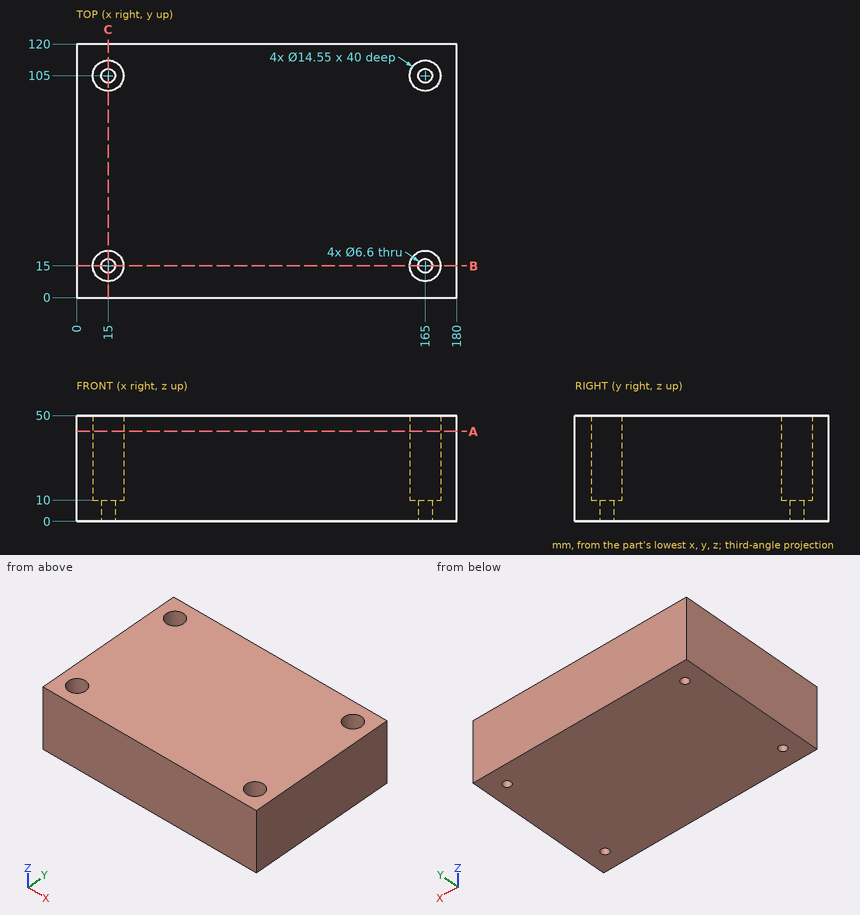
The drawing under review shows one solid part. Ordinate dimensions are in mm from its lowest x, y, z. Round coordinates to 2 decimals unless told otherwise and drop trailing zeros. Write each loop counter-clockwise with the first axis right and the second up, starting at its lowest first coordinate (ties: lowest second). Pieces come first, ordered by that corner, then holes. Notation, with made-up numbers: (2.25, 11) -> (40.25, 11) arc R25 ccw to (40.25, 41) -> close; hole circle Ø1 at (2, 17.25). An arc over 180 degrees is marked (long way). Put each result on its own line as item: value.
Q1. Clearance check with a flat-ended pin moving along its axis: pin 1 Ø4.5 at (x, y) = (15.5, 11.5) entering from +Z. State where the tip first meets the part, or that it passes through.
Determined:
pin 1: stops at z = 10
Q2. To check wall thickness, follow L1, parallel to Y at x = 15, z = 33 (3 decimals); L2, parallel to X at y = 15, z = 31.5 (3 decimals); L3, parallel to X at y = 105, z = 3.5. State the ranges of each line that lie inside material, in increasing order. Write a range as [from, to].
Determined:
L1: y = [0, 7.725], [22.275, 97.725], [112.275, 120]
L2: x = [0, 7.725], [22.275, 157.725], [172.275, 180]
L3: x = [0, 11.7], [18.3, 161.7], [168.3, 180]
Q3. Consider section B-B on y = 15. State the section outline as (x, z) points (3 decimals), and give its area (3 significant figures).
Determined:
outline: (0, 0) -> (11.7, 0) -> (11.7, 10) -> (7.725, 10) -> (7.725, 50) -> (0, 50) -> close; (18.3, 0) -> (161.7, 0) -> (161.7, 10) -> (157.725, 10) -> (157.725, 50) -> (22.275, 50) -> (22.275, 10) -> (18.3, 10) -> close; (168.3, 0) -> (180, 0) -> (180, 50) -> (172.275, 50) -> (172.275, 10) -> (168.3, 10) -> close
area: 7,700 mm^2
Q4. Consider section A-A on z = 42.5. State the section outline as (x, y) points (3 decimals), and give its area (3 significant figures).
Determined:
outline: (0, 0) -> (180, 0) -> (180, 120) -> (0, 120) -> close; hole circle Ø14.55 at (15, 15); hole circle Ø14.55 at (15, 105); hole circle Ø14.55 at (165, 15); hole circle Ø14.55 at (165, 105)
area: 20,900 mm^2
Q5. Consider section C-C on x = 15. State the section outline as (y, z) points (3 decimals).
Determined:
outline: (0, 0) -> (11.7, 0) -> (11.7, 10) -> (7.725, 10) -> (7.725, 50) -> (0, 50) -> close; (18.3, 0) -> (101.7, 0) -> (101.7, 10) -> (97.725, 10) -> (97.725, 50) -> (22.275, 50) -> (22.275, 10) -> (18.3, 10) -> close; (108.3, 0) -> (120, 0) -> (120, 50) -> (112.275, 50) -> (112.275, 10) -> (108.3, 10) -> close
